Autodesk Fusion 360 part; units mm, degrees
sketch "Sketch1" plane through (0, 0, 0) normal (0, 0, 1) x (1, 0, 0)
  circle A0 centre (0, 0) radius 8
  circle A1 centre (0, 0) radius 2.5
  circle A2 centre (0, 0) radius 6
  dimension "d1" = 16
  dimension "d2" = 5
  dimension "d3" = 12
extrude "Extrude1" add sketch "Sketch1" along normal blind 6.7 contours A0 | A2
extrude "Extrude2" add sketch "Sketch1" along normal blind 16 contours A2
extrude "Extrude3" add sketch "Sketch1" against normal blind 2 from surface at 16 contours A0
equation "d4 = 16 mm - 7.3 mm - 2 mm"
For this review, take the finished solid that the model builds, in its own axes (mm). A direction names the side the tool comes from. Round coordinates to 2 decimals unless told otherwise and drop trailing zeros. Loops run counter-clockwise (first coordinate to the right, second up) from the corner with the lowest first, then second, coordinate; pieces in that order, holes last. Notation, with made-up numbers: (0, -17.75) - (22, -17.75) arc R16 cw to (22, -0.75) - close; hole circle Ø1 at (22.5, 71.5). An arc over 180 degrees is marked (long way). Put each result on its own line as item: value. Start each with the question number.
1. Consider section A-A on y = 0. State the section outline as (x, z) points, plus the area to 3 significant figures.
2. Mouldability with a two-part tool opening along Z and no side actions: class faces 3 (the flat face through (-2, -2, 0)), 4 (the flat face through (-2, 6, 6.7)), 5 (the flat face through (-2, -2, 16)), 6 (the cylindrical face through (-1.73, -7.81, 15.01)) as +Z half, -Z half, draft (parallel to the pull), parting line (faces both ways), or undercut.
3. Consider section D-D on y = -5.25. State the section outline as (x, z) points, plus the area to 3 significant figures.
4. For probe 1 along Y at (x, z) = (0, 8.75); probe 2 along Y at (x, z) = (0, 6.5); probe 3 along Z at (x, y) = (5.75, 3.5), list the stretches that pass through material, from the lowest coordinate up. Write a range as [from, to].
5. Insertion check: P1, Ø3, axis at x = -5.5, z = 3, coming from the +Y side; P2, Ø1.5, axis at y = -6, z = 9, coming from the +X side; P3, Ø1, axis at x = 6, z = 2, coming from the +Y side. Each pin has a flat end and moves straight along its axis. Give the tip position at first contact, or say it passes through.
6. Consider section C-C on z = 9.5. State the section outline as (x, y) points, plus the area to 3 significant figures.
7. For faces 1 (the cylindrical face through (-0.54, 2.44, 7.89)), 2 (the flat face through (-2, 6, 14)), list the 3-axis set-ups (+Z, -Z, +X, -X, +Y, -Y) from which the entire face can be reached by the end or side of a thin tool; tool diameter is ignored.
Result sheet:
1. outline: (-8, 0) - (-2.5, 0) - (-2.5, 16) - (-8, 16) - (-8, 14) - (-6, 14) - (-6, 6.7) - (-8, 6.7) - close; (2.5, 0) - (8, 0) - (8, 6.7) - (6, 6.7) - (6, 14) - (8, 14) - (8, 16) - (2.5, 16) - close
1. area: 147 mm^2
2. face 3: -Z half
2. face 4: undercut
2. face 5: +Z half
2. face 6: draft
3. outline: (-6.04, 0) - (6.04, 0) - (6.04, 6.7) - (2.9, 6.7) - (2.9, 14) - (6.04, 14) - (6.04, 16) - (-6.04, 16) - (-6.04, 14) - (-2.9, 14) - (-2.9, 6.7) - (-6.04, 6.7) - close
3. area: 147 mm^2
4. probe 1: [-6, -2.5], [2.5, 6]
4. probe 2: [-8, -2.5], [2.5, 8]
4. probe 3: [0, 6.7], [14, 16]
5. P1: y = 6.93
5. P2: x = 2.9
5. P3: y = 5.81
6. outline: circle Ø12 at (0, 0); hole circle Ø5 at (0, 0)
6. area: 93.5 mm^2
7. face 1: +Z, -Z
7. face 2: none
